```python
from build123d import *

# Parameters (mm, degrees)
F0_W      = 56.0778109357
F0_H      = 53.2455928624
F1_DEPTH  = 44.704
F2_DEPTH  = 156.464
F3_W      = 24.2135291919
F3_H      = 31.2681160867
F4_DEPTH  = 49.276
F5_R      = 52.2926795061
F6_DEPTH  = 167.386
F7_W      = 28.2771997154
F7_H      = 13.4079456329
F8_DEPTH  = 34.29
F9_W      = 9.346306324
F9_H      = 19.2590444349
F10_DEPTH = 50.292
F11_W     = 10.2544277906
F11_H     = 16.5816796944
F12_DEPTH = 50.546
F13_W     = 28.7344292738
F13_H     = 8.3368938427
F14_DEPTH = 40.132
F15_DEPTH = 50.292
F16_W     = 56.0778109357
F16_H     = 53.2455928624
F17_DEPTH = 15.24
F18_R     = 14.2521119729
F19_DEPTH = 40.64


with BuildPart() as f1:
    # F0 (on Front) → F1 (new body)
    with BuildSketch(Plane.XZ):
        with Locations((18.1261622347, -3.8234870881)):
            Rectangle(F0_W, F0_H)
    extrude(amount=F1_DEPTH)

    # F2 (add): a face of the model
    f2_faces = [f1.faces().sort_by_distance(p)[0] for p in [
        (18.1261622347, 0, -3.8234870881),
    ]]
    extrude(f2_faces, amount=F2_DEPTH)

    # F3 (on face) → F4 (join)
    with BuildSketch(Plane.XY.offset(22.7993093431)):
        with Locations((20.3220699914, 15.6340580434)):
            Rectangle(F3_W, F3_H)
    extrude(amount=F4_DEPTH)

    # F5 (on face) → F6 (join)
    with BuildSketch(Plane.XZ.offset(44.704)):
        with Locations((18.975822255, 0)):
            Circle(F5_R)
    extrude(amount=-F6_DEPTH)

    # F7 (on face) → F8 (join)
    with BuildSketch(Plane.XY.offset(22.7993093431)):
        with Locations((14.1385998577, 136.814981699)):
            Rectangle(F7_W, F7_H)
    extrude(amount=F8_DEPTH)

    # F9 (on face) → F10 (join)
    with BuildSketch(Plane.YZ.offset(46.1650677025)):
        with Locations((137.4184936285, 5.2395930979)):
            Rectangle(F9_W, F9_H)
    extrude(amount=F10_DEPTH)

    # F11 (on face) → F12 (join)
    with BuildSketch(Plane(origin=(-9.9127432331, 0, 0), x_dir=(0, -1, 0), z_dir=(-1, 0, 0))):
        with Locations((-141.4983049035, 4.4673527591)):
            Rectangle(F11_W, F11_H)
    extrude(amount=F12_DEPTH)

    # F13 (on face) → F14 (join)
    with BuildSketch(Plane(origin=(0, 0, -30.4462835193), x_dir=(1, 0, 0), z_dir=(0, 0, -1))):
        with Locations((18.3513916563, -135.4045530787)):
            Rectangle(F13_W, F13_H)
    extrude(amount=F14_DEPTH)

    # F15 (add): a face of the model
    f15_faces = [f1.faces().sort_by_distance(p)[0] for p in [
        (-31.8377969197, 122.682, 0),
    ]]
    extrude(f15_faces, amount=F15_DEPTH)

    # F16 (on face) → F17 (join)
    with BuildSketch(Plane(origin=(0, 156.464, 0), x_dir=(-1, 0, 0), z_dir=(0, 1, 0))):
        with Locations((-18.1261622347, -3.8234870881)):
            Rectangle(F16_W, F16_H)
    extrude(amount=F17_DEPTH)

    # F18 (on face) → F19 (join)
    with BuildSketch(Plane(origin=(0, 171.704, 0), x_dir=(-1, 0, 0), z_dir=(0, 1, 0))):
        with Locations((-23.4041027725, 0)):
            Circle(F18_R)
    extrude(amount=F19_DEPTH)


solid = f1.part
```
Model file for the job. Use its own axes, mm. A direction names the side the tool comes from. Give positions to 0.01 mm unless a question says otherwise; leave off trailing zeros. Order: outer loops, then holes, each group sorted by start corner. A loop starts at its lowest first (then second) coordinate and runs counter-clockwise, first axis right, second up.
1) Saw through at C-C, the plane x = 76.5. Write the cut outline in (y, z).
2) Wall check: probe 1 along Y at (x, z) = (54, 36); probe 2 along X at (y, z) = (18, 2); probe 3 along Z at (x, y) = (-4, 130). Give the ranges that are in metal, low to high.
3) Saw through at B-B, the plane y = 8. Write the cut outline in (x, z), then the cut area to 3 significant figures.
4) Mould opens along Y. For faces 4 (the flat face through (14, 130.111, 54)), 5 (the flat face through (20, 31.268, 61)), 6 (the flat face through (-46, 136.371, 4)), 7 (the flat face through (96.457, 137, 5)) say: +Y half, -Y half, draft (parallel to the pull), parting line (faces both ways), or undercut.
5) 3-axis set-ups, long thin cutter, end or side, ignore diameter. For faces 1 (the flat face through (28.277, 137, 54)), 2 (the flat face through (14, 137, 57.089)), 3 (the flat face through (-46, 142, 12.758)): which of +Z, -Z, +X, -X, +Y, -Y reach the whole face in a straight line?
6) Saw through at A-A, the plane z = 0. Write the cut outline in (x, y).
7) Pin check, flat tips, straight feed: pin 1 (8 mm diameter, centred on x = -49, y = 143, fed in from -Z); pin 2 (10.5 mm diameter, centred on x = 89, y = 139, fed in from -Z); pin 3 (6 mm diameter, centred on x = 15, z = -58.5, fed in from -Y). Stop position of each tip, or through.
8) Saw through at D-D, the plane y = 165.5. Write the cut outline in (x, z), then the cut area to 3 significant figures.
Computed:
1. outline: (132.75, -4.39) - (142.09, -4.39) - (142.09, 14.87) - (132.75, 14.87) - close
2. probe 1: y = -44.7 to 172.97
2. probe 2: x = -33.28 to 71.23
2. probe 3: z = -46.97 to 46.97
3. outline: (8.22, 51.17) arc R52.29 ccw (long way) to (32.43, 50.53) - (32.43, 72.08) - (8.22, 72.08) - close
3. area: 9,080 mm2
4. face 4: undercut
4. face 5: undercut
4. face 6: -Y half
4. face 7: draft
5. face 1: +Z, +X, +Y
5. face 2: +Z, +X, -X, +Y
5. face 3: +Z, -X, +Y, -Y
6. outline: (-60.46, 136.37) - (-33.32, 136.37) - (-33.32, -44.7) - (71.27, -44.7) - (71.27, 132.75) - (96.46, 132.75) - (96.46, 142.09) - (71.27, 142.09) - (71.27, 172.97) - (46.17, 172.97) - (46.17, 171.7) - (37.66, 171.7) - (37.66, 212.34) - (9.15, 212.34) - (9.15, 171.7) - (-9.91, 171.7) - (-9.91, 172.97) - (-33.32, 172.97) - (-33.32, 146.63) - (-60.46, 146.63) - close
7. pin 1: stops at z = -3.82
7. pin 2: stops at z = -4.39
7. pin 3: stops at y = 131.24
8. outline: circle Ø104.59 at (18.98, 0)
8. area: 8,590 mm2
